Verification items for the finished model (mm, model axes). Round coordinates to 2 decimals unless told otherwise and drop trailing zeros. Write each loop counter-clockwise with the first axis right and the second up, starting at its lowest first coordinate (ties: lowest second). Pieces come first, ordered by that corner, then holes. Notation, with made-up numbers: M 41.25,16 L 45.25,16 A18 cw 45.25,35 Z; hole C 31.25,62 d10. An arc over 180 degrees is marked long. One line per item, written item: value. Start each with the question number.
from build123d import *

# Parameters (mm, degrees)
SKETCH1_R           = 8.5
BOSS_EXTRUDE1_DEPTH = 0.15
CUT_EXTRUDE1_REACH  = 2.3
SKETCH2_W           = 1
SKETCH2_H           = 9
SKETCH2_H_2         = 0.2


with BuildPart() as part:
    # Sketch1 → Boss-Extrude1 (new body, symmetric)
    with BuildSketch(Plane(origin=(0, 0, 0), x_dir=(1, 0, 0), z_dir=(0, 1, 0))):
        Circle(SKETCH1_R)
    extrude(amount=BOSS_EXTRUDE1_DEPTH, both=True)

    # Sketch2 → Cut-Extrude1 (cut, up to next)
    with BuildSketch(Plane(origin=(0, 0.15, 0), x_dir=(1, 0, 0), z_dir=(0, 1, 0)), mode=Mode.PRIVATE) as cut_extrude1_sk1:
        with Locations((0, 1.15)):
            Rectangle(SKETCH2_W, SKETCH2_H)
    cut_extrude1_tool1 = extrude(cut_extrude1_sk1.sketch, amount=-CUT_EXTRUDE1_REACH, mode=Mode.PRIVATE) & part.part
    add(cut_extrude1_tool1.solids().sort_by_distance((0, 0.15, -1.15))[0], mode=Mode.SUBTRACT)
    # Sketch2 → Cut-Extrude1 (cut, up to next)
    with BuildSketch(Plane(origin=(0, 0.15, 0), x_dir=(1, 0, 0), z_dir=(0, 1, 0)), mode=Mode.PRIVATE) as cut_extrude1_sk2:
        with Locations((4.5, -3.7)):
            Rectangle(SKETCH2_W, SKETCH2_H_2)
    cut_extrude1_tool2 = extrude(cut_extrude1_sk2.sketch, amount=-CUT_EXTRUDE1_REACH, mode=Mode.PRIVATE) & part.part
    add(cut_extrude1_tool2.solids().sort_by_distance((4.5, 0.15, 3.7))[0], mode=Mode.SUBTRACT)
    # Sketch2 → Cut-Extrude1 (cut, up to next)
    with BuildSketch(Plane(origin=(0, 0.15, 0), x_dir=(1, 0, 0), z_dir=(0, 1, 0)), mode=Mode.PRIVATE) as cut_extrude1_sk3:
        with Locations((-4.5, -3.7)):
            Rectangle(SKETCH2_W, SKETCH2_H_2)
    cut_extrude1_tool3 = extrude(cut_extrude1_sk3.sketch, amount=-CUT_EXTRUDE1_REACH, mode=Mode.PRIVATE) & part.part
    add(cut_extrude1_tool3.solids().sort_by_distance((-4.5, 0.15, 3.7))[0], mode=Mode.SUBTRACT)


solid = part.part
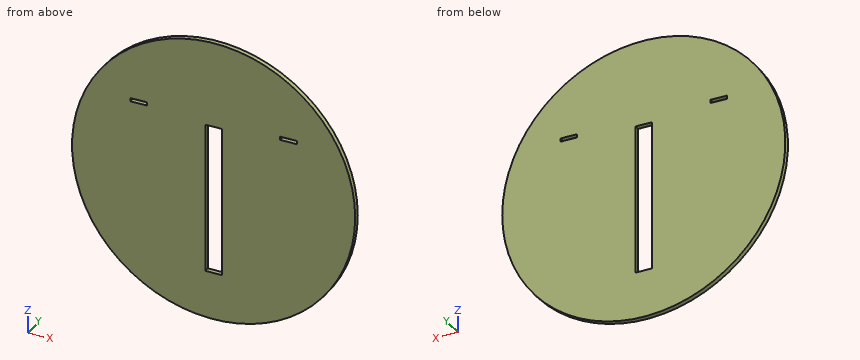
1) Thickness scan on line 1 (Z direction, x = 0.25, y = 0.1); line 2 (Z direction, x = -7.5, y = -0.1); line 3 (X direction, y = -0.1, z = 0.25). Record the ranges inside material, lowest first.
2) Cross-section at C-C (y = 0.05). Record the boundary of the cut face in (x, z).
3) Cross-section at D-D (x = 5.5). Record the boundary of the cut face in (y, z).
4) Cross-section at B-B (z = 0). Record the boundary of the cut face in (x, y).
5) Cross-section at A-A (x = 0). Record the boundary of the cut face in (y, z), then the cut area to 3 significant figures.
Results below:
1. line 1: z = -8.5 to -5.65, 3.35 to 8.5
1. line 2: z = -4 to 4
1. line 3: x = -8.5 to -0.5, 0.5 to 8.5
2. outline: C 0,0 d17; hole M -5,3.6 L -4,3.6 L -4,3.8 L -5,3.8 Z; hole M -0.5,-5.65 L 0.5,-5.65 L 0.5,3.35 L -0.5,3.35 Z; hole M 4,3.6 L 5,3.6 L 5,3.8 L 4,3.8 Z
3. outline: M -0.15,-6.48 L 0.15,-6.48 L 0.15,6.48 L -0.15,6.48 Z
4. outline: M -8.5,-0.15 L -0.5,-0.15 L -0.5,0.15 L -8.5,0.15 Z; M 0.5,-0.15 L 8.5,-0.15 L 8.5,0.15 L 0.5,0.15 Z
5. outline: M -0.15,-8.5 L 0.15,-8.5 L 0.15,-5.65 L -0.15,-5.65 Z; M -0.15,3.35 L 0.15,3.35 L 0.15,8.5 L -0.15,8.5 Z
5. area: 2.40 mm²
